CAD build for the part. Positions are in the model's coordinates, mm. Face numbers are marked on the shaded views. A direction names the side the tool comes from. Round coordinates to 2 decimals unless told otherwise and drop trailing zeros. Order: outer loops, then holes, each group sorted by start corner. A loop starts at its lowest first (then second) coordinate and runs counter-clockwise, first axis right, second up.
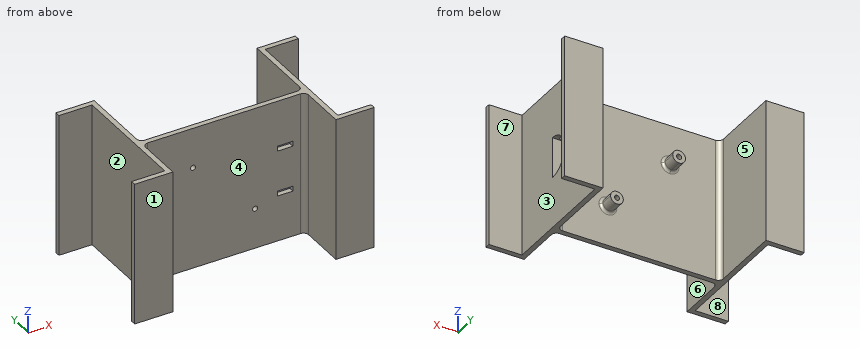
```python
from build123d import *

# Parameters (mm, degrees)
SKETCH1_W           = 2
SKETCH1_H           = 48
SKETCH1_W_2         = 64
SKETCH1_H_2         = 2
BOSS_EXTRUDE2_DEPTH = 56
BOSS_EXTRUDE3_DEPTH = 6
CUT_EXTRUDE1_START  = -31
SKETCH3_R           = 1
CUT_EXTRUDE1_DEPTH  = 31
SKETCH2_3_W         = 6
SKETCH2_3_H         = 2
CUT_EXTRUDE2_DEPTH  = 31
CUT_EXTRUDE3_DEPTH  = 31
FILLET1_R           = 1
FILLET2_R           = 2


with BuildPart() as part:
    # Sketch1 → Boss-Extrude2 (new body)
    with BuildSketch(Plane.XY):
        Polygon((-13, 48), (0, 48), (2, 48), (2, 50), (-13, 50), align=None)
        with Locations((1, 24)):
            Rectangle(SKETCH1_W, SKETCH1_H)
        Polygon((2, 0), (0, 0), (-13, 0), (-13, -2), (2, -2), align=None)
        with Locations((34, 19)):
            Rectangle(SKETCH1_W_2, SKETCH1_H_2)
        Polygon((66, 20), (66, 18), (66, 0), (68, 0), (68, 48), (66, 48), align=None)
        Polygon((68, 0), (66, 0), (66, -2), (81, -2), (81, 0), align=None)
        Polygon((66, 50), (66, 48), (68, 48), (81, 48), (81, 50), align=None)
    extrude(amount=BOSS_EXTRUDE2_DEPTH)

    # Sketch2 → Boss-Extrude3 (add)
    with BuildSketch(Plane(origin=(0, 20, 0), x_dir=(1, 0, 0), z_dir=(0, 1, 0))):
        with BuildLine():
            ThreePointArc((46.2, -16.8), (45.492893219, -16.507106781), (45.2, -15.8))
            Line((45.2, -15.8), (43.7, -15.8))
            ThreePointArc((43.7, -15.8), (44.432233047, -17.567766953), (46.2, -18.3))
            Line((46.2, -18.3), (46.2, -16.8))
        make_face()
        with BuildLine():
            Line((43.7, -15.8), (45.2, -15.8))
            ThreePointArc((45.2, -15.8), (46.2, -14.8), (47.2, -15.8))
            ThreePointArc((47.2, -15.8), (46.907106781, -16.507106781), (46.2, -16.8))
            Line((46.2, -16.8), (46.2, -18.3))
            ThreePointArc((46.2, -18.3), (47.967766953, -17.567766953), (48.7, -15.8))
            ThreePointArc((48.7, -15.8), (46.2, -13.3), (43.7, -15.8))
        make_face()
        with BuildLine():
            ThreePointArc((24.3, -40.2), (23.567766953, -38.432233047), (21.8, -37.7))
            Line((21.8, -37.7), (21.8, -39.2))
            ThreePointArc((21.8, -39.2), (22.507106781, -39.492893219), (22.8, -40.2))
            Line((22.8, -40.2), (24.3, -40.2))
        make_face()
        with BuildLine():
            Line((21.8, -39.2), (21.8, -37.7))
            ThreePointArc((21.8, -37.7), (20.032233047, -41.967766953), (24.3, -40.2))
            Line((24.3, -40.2), (22.8, -40.2))
            ThreePointArc((22.8, -40.2), (21.092893219, -40.907106781), (21.8, -39.2))
        make_face()
    extrude(amount=BOSS_EXTRUDE3_DEPTH)

    # Sketch3 → Cut-Extrude1 (cut)
    with BuildSketch(Plane(origin=(0, 20, 0), x_dir=(1, 0, 0), z_dir=(0, 1, 0)).offset(CUT_EXTRUDE1_START)):
        with Locations(Location((46.2, -15.8, 0), (0, 0, 270))):
            Circle(SKETCH3_R)
        with Locations(Location((21.8, -40.2, 0), (0, 0, 270))):
            Circle(SKETCH3_R)
    extrude(amount=CUT_EXTRUDE1_DEPTH, mode=Mode.SUBTRACT)

    # Sketch2_3 → Cut-Extrude2 (cut)
    with BuildSketch(Plane(origin=(0, 20, 0), x_dir=(1, 0, 0), z_dir=(0, 1, 0))):
        with Locations((58, -19)):
            Rectangle(SKETCH2_3_W, SKETCH2_3_H)
        with Locations((58, -37)):
            Rectangle(SKETCH2_3_W, SKETCH2_3_H)
    extrude(amount=-CUT_EXTRUDE2_DEPTH, mode=Mode.SUBTRACT)

    # Sketch6 → Cut-Extrude3 (cut)
    with BuildSketch(Plane.ZY.offset(-66)):
        with BuildLine():
            Line((35.999989218, 20), (20.000010782, 20))
            ThreePointArc((20.000010782, 20), (28, 27.999989218), (35.999989218, 20))
        make_face()
    extrude(amount=-CUT_EXTRUDE3_DEPTH, mode=Mode.SUBTRACT)

    # Fillet1
    fillet1_edges = [part.edges().sort_by_distance(p)[0] for p in [
        (48.7, 20, 15.8),
        (19.3, 20, 40.2),
    ]]
    fillet(fillet1_edges, radius=FILLET1_R)

    # Fillet2
    fillet2_edges = [part.edges().sort_by_distance(p)[0] for p in [
        (66, 20, 10.000005391),
        (2, 20, 28),
        (66, 20, 45.999994609),
        (66, 18, 28),
        (2, 18, 28),
    ]]
    fillet(fillet2_edges, radius=FILLET2_R)


solid = part.part
```
1. Pin check, flat tips, straight feed: P1, Ø9, axis at y = 6.5, z = 29, coming from the -X side; P2, Ø1, axis at x = 53.5, z = 17.5, coming from the -Y side; P3, Ø4, axis at x = 47.5, z = 17, coming from the +Y side. Stop position of each tip, or through.
2. Cut at A-A, the plane z = 28. Write the cut outline in (x, y), and give its area (3 significant figures).
3. Cut at C-C, the plane z = 10. Write the cut outline in (x, y).
4. Drill centre lines: line 1 (X direction, y = 24.4, z = 40.2); line 2 (X direction, y = 30.5, z = 19); line 3 (Z direction, x = 21.8, y = 18.75). Where is each one in solid material? Low to high.
5. Mould opens along X. For the marked faces 1, 2, 3 and 4 say: released by +X, released by -X, zero draft, split by the parting line, or undercut.
6. Tool access for the marked faces 5, 6, 7 and 8: list every direction of +Z, -Z, +X, -X, +Y, -Y with a clear straight run to the whole face (end or side of a thin tool).
7. Cut at D-D, the plane y = 23. Write the cut outline in (x, z), and give its area (3 significant figures).
8. Cut at B-B, the plane y = 45. Write the cut outline in (x, z), and give its area (3 significant figures).
Outcome:
1. P1: stops at x = 0
1. P2: stops at y = 18
1. P3: stops at y = 26
2. outline: (-13, -2) - (2, -2) - (2, 16) arc R2 cw to (4, 18) - (64, 18) arc R2 cw to (66, 16) - (66, -2) - (81, -2) - (81, 0) - (68, 0) - (68, 20) - (4, 20) arc R2 cw to (2, 22) - (2, 50) - (-13, 50) - (-13, 48) - (0, 48) - (0, 0) - (-13, 0) - close; (66, 28) - (68, 28) - (68, 48) - (81, 48) - (81, 50) - (66, 50) - close
2. area: 427 mm2
3. outline: (-13, -2) - (2, -2) - (2, 16) arc R2 cw to (4, 18) - (64, 18) arc R2 cw to (66, 16) - (66, -2) - (81, -2) - (81, 0) - (68, 0) - (68, 48) - (81, 48) - (81, 50) - (66, 50) - (66, 22) arc R2 cw to (64, 20) - (4, 20) arc R2 cw to (2, 22) - (2, 50) - (-13, 50) - (-13, 48) - (0, 48) - (0, 0) - (-13, 0) - close
4. line 1: x = 0 to 2, 19.3 to 20.8, 22.8 to 24.3, 66 to 68
4. line 2: x = 0 to 2, 66 to 68
4. line 3: z = 0 to 39.2, 41.2 to 56
5. face 1: zero draft
5. face 2: released by -X
5. face 3: released by +X
5. face 4: undercut
6. face 5: +Z, -Z, +Y
6. face 6: +Z, -Z, -Y
6. face 7: +Z, -Z, +X
6. face 8: +Z, -Z, -X
7. outline: (0, 0) - (2, 0) - (2, 56) - (0, 56) - close; circle Ø5 at (21.8, 40.2); circle Ø5 at (46.2, 15.8); (66, 0) - (68, 0) - (68, 20.58) - (66, 20.58) - close; (66, 35.42) - (68, 35.42) - (68, 56) - (66, 56) - close; hole circle Ø2 at (21.8, 40.2); hole circle Ø2 at (46.2, 15.8)
7. area: 227 mm2
8. outline: (0, 0) - (2, 0) - (2, 56) - (0, 56) - close; (66, 0) - (68, 0) - (68, 56) - (66, 56) - close
8. area: 224 mm2
